```python
from build123d import *

# Parameters (mm, degrees)
F1_DEPTH = 750
F3_DEPTH = 25


with BuildPart() as f1:
    # F0 (on Front) → F1 (new body)
    with BuildSketch(Plane.XZ):
        Polygon((5.032131, -5.975653), (-16.967869, -5.975653), (-16.967869, -8.975653), (8.032131, -8.975653), (8.032131, 16.024347), (5.032131, 16.024347), align=None)
    extrude(amount=F1_DEPTH)

    # F2 (on face) → F3 (cut)
    with BuildSketch(Plane(origin=(0, 0, -8.975653), x_dir=(1, 0, 0), z_dir=(0, 0, -1))):
        Polygon((8.032131, 750), (-16.967869, 750), (8.032131, 725), align=None)
    extrude(amount=-F3_DEPTH, mode=Mode.SUBTRACT)


with BuildPart() as f4_1:
    # F4: instance of F1
    add(f1.part.mirror(Plane.XZ))


solid = f4_1.part
```
Model file for the job. Use its own axes, mm. A direction names the side the tool comes from. Give positions to 0.01 mm unless a question says otherwise; leave off trailing zeros. Loops run counter-clockwise (first coordinate to the right, second up) from the corner with the lowest first, then second, coordinate; pieces in that order, holes last. Notation, with made-up numbers: M 15,51 L 23,51 A18 ccw 23,56 Z; hole C -11.5,89 d11. An arc over 180 degrees is marked long. Use one line per item in the form item = value.
Item 1: Flat gauge pins, fed straight in: pin 1 Ø6.5 at (x, y) = (-8, 195.5) entering from +Z; pin 2 Ø10 at (x, z) = (5.5, 12.5) entering from -Y. Where does each tip first touch, or does it go through?
Filled in:
pin_1 = -5.98
pin_2 = 0
Item 2: Slice it at C-C on z = -1. List the corners of the cut face in (x, y).
Filled in:
outline = M 5.03,0 L 8.03,0 L 8.03,725 L 5.03,728 Z
Item 3: Slice it at A-A on y = 150. List the corners of the cut face in (x, z).
Filled in:
outline = M -16.97,-8.98 L 8.03,-8.98 L 8.03,16.02 L 5.03,16.02 L 5.03,-5.98 L -16.97,-5.98 Z
Item 4: Slice it at B-B on x = -11.5. List the corners of the cut face in (y, z), and give its area (3 significant figures).
Filled in:
outline = M 0,-8.98 L 744.53,-8.98 L 744.53,-5.98 L 0,-5.98 Z
area = 2,230 mm^2
Item 5: Which spindle directions (+Z, -Z, +X, -X, +Y, -Y) get a long thin tool onto all of the face, cutting with end or side? Do faces 1 (the flat face through (-6, 370, -5.976)), 2 (the flat face through (8.032, 357, 3)). Say none if no direction does.
Filled in:
face_1 = +Z, -X, +Y, -Y
face_2 = +Z, -Z, +X, +Y, -Y
Item 6: Drill centre lines: L1, parallel to Z at x = -0.75, y = 614; L2, parallel to X at y = 672, z = 14.5; L3, parallel to Y at x = -9, z = -6.25. Where is each one in solid material? Low to high.
Filled in:
L1 = -8.98 to -5.98
L2 = 5.03 to 8.03
L3 = 0 to 742.03
